from build123d import *

# Parameters (mm, degrees)
BOSS_EXTRUDE1_DEPTH = 24.13
BOSS_EXTRUDE2_DEPTH = 5.08
LPATTERN1_COUNT     = 2
LPATTERN1_PITCH     = 53.34
FILLET1_R           = 5.08


with BuildPart() as part:
    # Sketch1 → Boss-Extrude1 (new, symmetric)
    with BuildSketch(Plane.XY):
        with BuildLine():
            Line((-25.527, 0), (25.527, 0))
            Line((25.527, 0), (25.527, -25.654))
            Line((25.527, -25.654), (23.749, -25.654))
            Line((23.749, -25.654), (23.749, -29.464))
            Line((23.749, -29.464), (29.337, -29.464))
            Line((29.337, -29.464), (29.337, 3.81))
            ThreePointArc((29.337, 3.81), (0, 13.137353219), (-29.337, 3.81))
            Line((-29.337, 3.81), (-29.337, -29.464))
            Line((-29.337, -29.464), (-23.749, -29.464))
            Line((-23.749, -29.464), (-23.749, -25.654))
            Line((-23.749, -25.654), (-25.527, -25.654))
            Line((-25.527, -25.654), (-25.527, 0))
        make_face()
    extrude(amount=BOSS_EXTRUDE1_DEPTH, both=True)

    # Sketch2 → Boss-Extrude2 (add)
    with BuildSketch(Plane.XY.offset(24.13)):
        with BuildLine():
            Line((29.337, -29.464), (29.337, 8.89))
            ThreePointArc((29.337, 8.89), (0, 18.217353219), (-29.337, 8.89))
            Line((-29.337, 8.89), (-29.337, -29.464))
            Line((-29.337, -29.464), (-23.749, -29.464))
            Line((-23.749, -29.464), (-23.749, -25.654))
            Line((-23.749, -25.654), (-25.527, -25.654))
            Line((-25.527, -25.654), (-25.527, 0))
            Line((-25.527, 0), (25.527, 0))
            Line((25.527, 0), (25.527, -25.654))
            Line((25.527, -25.654), (23.749, -25.654))
            Line((23.749, -25.654), (23.749, -29.464))
            Line((23.749, -29.464), (29.337, -29.464))
        make_face()
    boss_extrude2 = extrude(amount=BOSS_EXTRUDE2_DEPTH)

    # LPattern1: Boss-Extrude2 ×2
    with Locations(*[(0, 0, -i * LPATTERN1_PITCH) for i in range(1, LPATTERN1_COUNT)]):
        add(boss_extrude2)

    # Fillet1
    fillet1_edges = [part.edges().sort_by_distance(p)[0] for p in [
        (-29.337, 3.81, 0),
        (29.337, 3.81, 0),
        (29.337, 8.89, 26.67),
        (-29.337, 8.89, 26.67),
        (29.337, 8.89, -26.67),
        (-29.337, 8.89, -26.67),
    ]]
    fillet(fillet1_edges, radius=FILLET1_R)


solid = part.part
CAD build for the part. Positions are in the model's coordinates, mm. A direction names the side the tool comes from. Coordinates: 2 decimals unless noted, no trailing zeros. Order: outer loops, then holes, each group sorted by start corner. A loop starts at its lowest first (then second) coordinate and runs counter-clockwise, first axis right, second up. Notation, with made-up numbers: (23.5, -24.5) -> (58.5, -24.5) arc R20 cw to (58.5, -5.5) -> close; hole circle Ø8 at (-34.5, 36.5). An arc over 180 degrees is marked (long way). Answer in a Markdown table with one row per item.
1) Flat gauge pins, fed straight in: P1, Ø1, axis at x = 18, z = 2, coming from the -Y side; P2, Ø2, axis at x = -24.5, z = 14, coming from the +Y side (3 decimals); P3, Ø6, axis at x = 13, z = -20, coming from the +Y side. Where does each tip first touch, or does it go through?
Check values:
| item | result |
|---|---|
| P1 | y = 0 |
| P2 | y = 7.375 |
| P3 | y = 12.14 |
2) Mould opens along Z. For faces 1 (the face through (27, -29.464, 0)), 2 (the face through (0.398, 13.136, 0.338)), 3 (the face through (0, 5, 29.21)) say: pulls with the +Z half, pulls with the -Z half, needs draft (parallel to the pull), parting line crosses it, or undercut.
Check values:
| item | result |
|---|---|
| face 1 | needs draft |
| face 2 | undercut |
| face 3 | pulls with the +Z half |
3) Band-saw the part on A-A (y = -23). List the corners of the cut face in (x, z), and give its area (3 significant figures).
Check values:
| item | result |
|---|---|
| outline | (-29.34, -29.21) -> (-25.53, -29.21) -> (-25.53, 29.21) -> (-29.34, 29.21) -> close; (25.53, -29.21) -> (29.34, -29.21) -> (29.34, 29.21) -> (25.53, 29.21) -> close |
| area | 445 mm2 |
4) Band-saw the part on C-C (z = -14). List the corners of the cut face in (x, y).
Check values:
| item | result |
|---|---|
| outline | (-29.34, -29.46) -> (-23.75, -29.46) -> (-23.75, -25.65) -> (-25.53, -25.65) -> (-25.53, 0) -> (25.53, 0) -> (25.53, -25.65) -> (23.75, -25.65) -> (23.75, -29.46) -> (29.34, -29.46) -> (29.34, 1.09) arc R5.08 ccw to (26.95, 5.4) arc R50.8 ccw to (-26.95, 5.4) arc R5.08 ccw to (-29.34, 1.09) -> close |
5) Band-saw the part on B-B (x = 15.5). List the corners of the cut face in (y, z).
Check values:
| item | result |
|---|---|
| outline | (0, -29.21) -> (15.79, -29.21) -> (15.79, -24.13) -> (10.71, -24.13) -> (10.71, 24.13) -> (15.79, 24.13) -> (15.79, 29.21) -> (0, 29.21) -> close |
6) Drill centre lines: line 1 (X direction, y = -23, z = 0); line 2 (Z direction, x = 18, y = 10); line 3 (Y direction, x = 0, z = -6). Where is each one in solid material? Low to high.
Check values:
| item | result |
|---|---|
| line 1 | -29.34 to -25.53, 25.53 to 29.34 |
| line 2 | -29.21 to -24.13, 24.13 to 29.21 |
| line 3 | 0 to 13.14 |
7) Which spindle directions (+Z, -Z, +X, -X, +Y, -Y) get a long thin tool onto all of the face, cutting with end or side? Do faces 4 (the face through (0, 15, 24.13)), 5 (the face through (28.72, 3.52, 0.34)), 6 (the face through (-25, -25.654, 0)). Say none if no direction does.
Check values:
| item | result |
|---|---|
| face 4 | +Y |
| face 5 | +X, +Y |
| face 6 | +Z, -Z |
8) Band-saw the part on D-D (y = 3.5). List the corners of the cut face in (x, z), and give its area (3 significant figures).
Check values:
| item | result |
|---|---|
| outline | (-29.34, -29.21) -> (29.34, -29.21) -> (29.34, -24.13) -> (28.73, -24.13) -> (28.73, 24.13) -> (29.34, 24.13) -> (29.34, 29.21) -> (-29.34, 29.21) -> (-29.34, 24.13) -> (-28.73, 24.13) -> (-28.73, -24.13) -> (-29.34, -24.13) -> close |
| area | 3,370 mm2 |
